Input: part model. Units: mm. Frame: model coordinates. Coordinates: 2 decimals unless noted, no trailing zeros. Write each loop counter-clockwise with the first axis right and the second up, starting at its lowest first coordinate (ties: lowest second). Pieces come first, ordered by that corner, then holes.
1) Pin query (flat end, axial travel): pin 1 Ø1.5 at (y, z) = (76, 1.5) entering from +X. Return the tip coordinate at first contact, or that it passes through.
2) Section query A-A (z = 1.05). State how many separate pieces and enclosed holes the cut face has, then the cut area to 3 significant figures.
3) Draft query along Y for faces 1 (the cylindrical face through (-76.925, 82.686, 1.521)), 2 (the flat face through (-1, 1, 0)). Return one class per face: pulls with the +Y half, pulls with the -Y half, needs draft (parallel to the pull), parting line crosses it, or undercut.
4) Line query: L1, parallel to X at y = -86, z = 1.4; L2, parallel to Y at x = -84, z = 2.35; L3, parallel to Y at x = -78, z = 0.6. Output: solid intervals per line, ascending.
5) Section query B-B (y = 42.5). Output: boundary loops of the cut face in (x, z), then the cut area to 3 significant figures.
6) Section query C-C (x = 69). Output: boundary loops of the cut face in (y, z), then the cut area to 3 significant figures.
Autodesk Inventor part; units mm, degrees
ref_plane "YZ Plane" through (0, 0, 0) normal (1, 0, 0) x (0, 1, 0)
ref_plane "XZ Plane" through (0, 0, 0) normal (0, 1, 0) x (-1, 0, 0)
ref_plane "XY Plane" through (0, 0, 0) normal (0, 0, 1) x (1, 0, 0)
sketch "Sketch1" plane through (0, 0, 0) normal (0, 0, 1) x (1, 0, 0)
  line L0 (-90.5, -90.5) -> (90.5, -90.5)
  line L1 (90.5, -90.5) -> (90.5, 90.5)
  line L2 (90.5, 90.5) -> (-90.5, 90.5)
  line L3 (-90.5, 90.5) -> (-90.5, -90.5)
  line L4 (-90.5, -90.5) -> (90.5, 90.5) construction
  line L5 (90.5, -90.5) -> (-90.5, 90.5) construction
  point P0 (0, 0)
  dimension "d0" = 181
  dimension "d1" = 181
extrude "Extrusion1" add sketch "Sketch1" along normal blind 3
sketch "Sketch2" plane through (0, 0, 3) normal (0, 0, 1) x (1, 0, 0)
  line L0 (90.5, 90.5) -> (-90.5, 90.5)
  line L1 (-90.5, 90.5) -> (-85, 90.5)
  line L2 (-85, 90.5) -> (-85, 93.5)
  line L3 (-85, 93.5) -> (-90.5, 93.5)
  line L4 (-90.5, 93.5) -> (-90.5, 90.5)
  line L5 (80, 90.5) -> (85.5, 90.5)
  line L6 (85.5, 90.5) -> (85.5, 93.5)
  line L7 (85.5, 93.5) -> (80, 93.5)
  line L8 (80, 93.5) -> (80, 90.5)
  line L9 (-90.5, -93.5) -> (-85, -93.5)
  line L10 (-85, -93.5) -> (-85, -90.5)
  line L11 (-85, -90.5) -> (-90.5, -90.5)
  line L12 (-90.5, -90.5) -> (-90.5, -93.5)
  line L13 (80, -93.5) -> (85.5, -93.5)
  line L14 (85.5, -93.5) -> (85.5, -90.5)
  line L15 (85.5, -90.5) -> (80, -90.5)
  line L16 (80, -90.5) -> (80, -93.5)
  line L17 (-70, 90.5) -> (-55, 90.5)
  line L18 (-55, 90.5) -> (-55, 93.5)
  line L19 (-55, 93.5) -> (-70, 93.5)
  line L20 (-70, 93.5) -> (-70, 90.5)
  line L21 (-25, 90.5) -> (-25, 93.5)
  line L22 (-40, 90.5) -> (-25, 90.5)
  line L23 (-25, 93.5) -> (-40, 93.5)
  line L24 (-40, 93.5) -> (-40, 90.5)
  line L25 (5, 90.5) -> (5, 93.5)
  line L26 (-10, 90.5) -> (5, 90.5)
  line L27 (5, 93.5) -> (-10, 93.5)
  line L28 (-10, 93.5) -> (-10, 90.5)
  line L29 (35, 90.5) -> (35, 93.5)
  line L30 (20, 90.5) -> (35, 90.5)
  line L31 (35, 93.5) -> (20, 93.5)
  line L32 (20, 93.5) -> (20, 90.5)
  line L33 (65, 90.5) -> (65, 93.5)
  line L34 (50, 90.5) -> (65, 90.5)
  line L35 (65, 93.5) -> (50, 93.5)
  line L36 (50, 93.5) -> (50, 90.5)
  line L37 (-55, -93.5) -> (-55, -90.5)
  line L38 (-70, -93.5) -> (-55, -93.5)
  line L39 (-55, -90.5) -> (-70, -90.5)
  line L40 (-70, -90.5) -> (-70, -93.5)
  line L41 (-25, -93.5) -> (-25, -90.5)
  line L42 (-40, -93.5) -> (-25, -93.5)
  line L43 (-25, -90.5) -> (-40, -90.5)
  line L44 (-40, -90.5) -> (-40, -93.5)
  line L45 (5, -93.5) -> (5, -90.5)
  line L46 (-10, -93.5) -> (5, -93.5)
  line L47 (5, -90.5) -> (-10, -90.5)
  line L48 (-10, -90.5) -> (-10, -93.5)
  line L49 (35, -93.5) -> (35, -90.5)
  line L50 (20, -93.5) -> (35, -93.5)
  line L51 (35, -90.5) -> (20, -90.5)
  line L52 (20, -90.5) -> (20, -93.5)
  line L53 (65, -93.5) -> (65, -90.5)
  line L54 (50, -93.5) -> (65, -93.5)
  line L55 (65, -90.5) -> (50, -90.5)
  line L56 (50, -90.5) -> (50, -93.5)
  point P0 (0, 0)
  dimension "d4" = 5.5
  dimension "d5" = 3
  dimension "d8" = 170.5
  dimension "d11" = 184
  dimension "d14" = 15
  dimension "d15" = 3
  dimension "d16" = 15
  dimension "d19" = 30
  dimension "d22" = 184
extrude "Extrusion2" add sketch "Sketch2" against normal blind 3
sketch "Sketch3" plane through (0, 0, 3) normal (0, 0, 1) x (1, 0, 0)
  line L0 (-90.5, 93.5) -> (-90.5, -93.5)
  line L1 (-90.5, 82.5) -> (-87.5, 82.5)
  line L2 (-87.5, 82.5) -> (-87.5, 67.5)
  line L3 (-87.5, 67.5) -> (-90.5, 67.5)
  line L4 (-90.5, 67.5) -> (-90.5, 82.5)
  line L5 (-85, 93.5) -> (-90.5, 93.5)
  line L6 (-90.5, 52.5) -> (-87.5, 52.5)
  line L7 (-87.5, 52.5) -> (-87.5, 37.5)
  line L8 (-87.5, 37.5) -> (-90.5, 37.5)
  line L9 (-90.5, 37.5) -> (-90.5, 52.5)
  line L10 (-90.5, 22.5) -> (-87.5, 22.5)
  line L11 (-87.5, 22.5) -> (-87.5, 7.5)
  line L12 (-87.5, 7.5) -> (-90.5, 7.5)
  line L13 (-90.5, 7.5) -> (-90.5, 22.5)
  line L14 (-90.5, -7.5) -> (-87.5, -7.5)
  line L15 (-87.5, -7.5) -> (-87.5, -22.5)
  line L16 (-87.5, -22.5) -> (-90.5, -22.5)
  line L17 (-90.5, -22.5) -> (-90.5, -7.5)
  line L18 (-90.5, -37.5) -> (-87.5, -37.5)
  line L19 (-87.5, -37.5) -> (-87.5, -52.5)
  line L20 (-87.5, -52.5) -> (-90.5, -52.5)
  line L21 (-90.5, -52.5) -> (-90.5, -37.5)
  line L22 (-90.5, -67.5) -> (-87.5, -67.5)
  line L23 (-87.5, -67.5) -> (-87.5, -82.5)
  line L24 (-87.5, -82.5) -> (-90.5, -82.5)
  line L25 (-90.5, -82.5) -> (-90.5, -67.5)
  line L26 (87.5, 82.5) -> (90.5, 82.5)
  line L27 (90.5, 82.5) -> (90.5, 67.5)
  line L28 (90.5, 67.5) -> (87.5, 67.5)
  line L29 (87.5, 67.5) -> (87.5, 82.5)
  line L30 (87.5, 52.5) -> (90.5, 52.5)
  line L31 (90.5, 52.5) -> (90.5, 37.5)
  line L32 (90.5, 37.5) -> (87.5, 37.5)
  line L33 (87.5, 37.5) -> (87.5, 52.5)
  line L34 (87.5, 22.5) -> (90.5, 22.5)
  line L35 (90.5, 22.5) -> (90.5, 7.5)
  line L36 (90.5, 7.5) -> (87.5, 7.5)
  line L37 (87.5, 7.5) -> (87.5, 22.5)
  line L38 (87.5, -7.5) -> (90.5, -7.5)
  line L39 (90.5, -7.5) -> (90.5, -22.5)
  line L40 (90.5, -22.5) -> (87.5, -22.5)
  line L41 (87.5, -22.5) -> (87.5, -7.5)
  line L42 (87.5, -37.5) -> (90.5, -37.5)
  line L43 (90.5, -37.5) -> (90.5, -52.5)
  line L44 (90.5, -52.5) -> (87.5, -52.5)
  line L45 (87.5, -52.5) -> (87.5, -37.5)
  line L46 (87.5, -67.5) -> (90.5, -67.5)
  line L47 (90.5, -67.5) -> (90.5, -82.5)
  line L48 (90.5, -82.5) -> (87.5, -82.5)
  line L49 (87.5, -82.5) -> (87.5, -67.5)
  point P0 (0, 0)
  dimension "d27" = 3
  dimension "d28" = 15
  dimension "d29" = 11
  dimension "d32" = 30
  dimension "d35" = 178
extrude "Extrusion3" cut sketch "Sketch3" against normal blind 3
sketch "Sketch4" plane through (0, 0, 3) normal (0, 0, 1) x (1, 0, 0)
  line L0 (80, 93.5) -> (85.5, 93.5)
  line L1 (90.5, 90.5) -> (85.5, 90.5)
  line L2 (85.5, 93.5) -> (90.5, 93.5)
  line L3 (90.5, 93.5) -> (90.5, 90.5)
  line L4 (90.5, 90.5) -> (85.5, 90.5)
  line L5 (85.5, 90.5) -> (85.5, 93.5)
  line L6 (85.5, -90.5) -> (90.5, -90.5)
  line L7 (85.5, -90.5) -> (90.5, -90.5)
  line L8 (90.5, -90.5) -> (90.5, -93.5)
  line L9 (90.5, -93.5) -> (85.5, -93.5)
  line L10 (85.5, -93.5) -> (85.5, -90.5)
  point P0 (0, 0)
  dimension "d40" = 184
extrude "Extrusion4" add sketch "Sketch4" against normal blind 3
sketch "Sketch5" plane through (0, 0, 3) normal (0, 0, 1) x (1, 0, 0)
  circle A0 centre (-84, -86) radius 1.5
  circle A1 centre (84, -86) radius 1.5
  line L0 (90.5, -82.5) -> (90.5, -93.5)
  line L1 (90.5, -93.5) -> (80, -93.5)
  line L2 (-85, -93.5) -> (-90.5, -93.5)
  line L3 (-90.5, -82.5) -> (-90.5, -93.5)
  point P0 (0, 0)
  dimension "d43" = 3
  dimension "d44" = 3
  dimension "d45" = 6.5
  dimension "d46" = 7.5
  dimension "d47" = 7.5
  dimension "d48" = 6.5
extrude "Extrusion5" cut sketch "Sketch5" against normal blind 10
sketch "Sketch6" plane through (0, 0, 3) normal (0, 0, 1) x (1, 0, 0)
  circle A0 centre (-78, 81) radius 2
  circle A1 centre (78, 81) radius 2
  line L0 (-87.5, 82.5) -> (-87.5, 67.5)
  line L1 (-70, 90.5) -> (-85, 90.5)
  line L2 (80, 90.5) -> (65, 90.5)
  line L3 (87.5, 67.5) -> (87.5, 82.5)
  point P0 (0, 0)
  dimension "d51" = 4
  dimension "d52" = 4
  dimension "d53" = 9.5
  dimension "d54" = 9.5
  dimension "d55" = 9.5
  dimension "d56" = 9.5
extrude "Extrusion6" cut sketch "Sketch6" against normal blind 10
equation "\"d47\" = d46"
equation "\"d48\" = d45"
equation "\"BendRadius\" = Thickness"
equation "\"BendReliefWidth\" = Thickness"
equation "\"BendReliefDepth\" = 0.5 * Thickness"
equation "\"CornerReliefSize\" = 4 * Thickness"
equation "\"MinimumRemnant\" = 2 * Thickness"
equation "\"TransitionRadius\" = BendRadius"
equation "\"JacobiRadiusSize\" = BendRadius"
equation "\"GapSize\" = Thickness"
properties part number "7 achter plaat"
Answer:
1. pin 1: stops at x = 87.5
2. separate pieces: 1
2. enclosed holes: 4
2. area: 32,700 mm2
3. face 1: undercut
3. face 2: needs draft
4. L1: x = -90.5 to -85.5, -82.5 to 82.5, 85.5 to 90.5
4. L2: y = -90.5 to -87.5, -84.5 to 90.5
4. L3: y = -90.5 to 79, 83 to 90.5
5. outline: (-87.5, 0) - (87.5, 0) - (87.5, 3) - (-87.5, 3) - close
5. area: 525 mm2
6. outline: (-90.5, 0) - (90.5, 0) - (90.5, 3) - (-90.5, 3) - close
6. area: 543 mm2
